```python
from build123d import *

# Parameters (mm, degrees)
SKETCH1_W           = 30
SKETCH1_H           = 13.3
BOSS_EXTRUDE1_DEPTH = 10.75
SKETCH2_W           = 8
SKETCH2_H           = 4.6
CUT_EXTRUDE1_DEPTH  = 6
FILLET1_R           = 0.2


with BuildPart() as part:
    # Sketch1 → Boss-Extrude1 (new body)
    with BuildSketch(Plane.XY):
        Rectangle(SKETCH1_W, SKETCH1_H)
    extrude(amount=BOSS_EXTRUDE1_DEPTH)

    # Sketch2 → Cut-Extrude1 (cut)
    with BuildSketch(Plane(origin=(15, 0, 0), x_dir=(0, 0, -1), z_dir=(1, 0, 0))):
        with Locations((-6.75, -3)):
            Rectangle(SKETCH2_W, SKETCH2_H)
        with Locations((-6.75, 3)):
            Rectangle(SKETCH2_W, SKETCH2_H)
    extrude(amount=-CUT_EXTRUDE1_DEPTH, mode=Mode.SUBTRACT)

    # Fillet1
    fillet1_edges = [part.edges().sort_by_distance(p)[0] for p in [
        (15, -5.975, 10.75),
        (15, 0, 10.75),
        (15, 5.975, 10.75),
        (0, 6.65, 10.75),
        (-15, 0, 10.75),
        (0, 6.65, 0),
        (15, 0, 0),
        (0, -6.65, 0),
        (-15, 0, 0),
        (-15, 6.65, 5.375),
        (15, 6.65, 5.375),
        (15, -6.65, 5.375),
        (-15, -6.65, 5.375),
        (0, -6.65, 10.75),
    ]]
    fillet(fillet1_edges, radius=FILLET1_R)


solid = part.part
```
Source: CAD feature listing. Evaluate the final solid. Frame: model axes, mm. A direction names the side the tool comes from. Give positions to 0.01 mm unless a question says otherwise; leave off trailing zeros. Loops run counter-clockwise (first coordinate to the right, second up) from the corner with the lowest first, then second, coordinate; pieces in that order, holes last. Notation, with made-up numbers: (89, 73) - (134, 73) arc R21 cw to (134, 84) - close; hole circle Ø6 at (80.5, 17.5). An arc over 180 degrees is marked (long way). Use CSV: the item, a comma, the result in double quotes. Start each with the question number.
1. Draft query along Y for faces 3 (the flat face through (15, 0, 4)), 4 (the flat face through (0, 6.65, 5)), 5 (the flat face through (12, 5.3, 7)). Return one class per face: +Y half, -Y half, draft (parallel to the pull), parting line (faces both ways), or undercut.
2. Section A-A (x = 10.5). Output: boundary loops of the cut face in (y, z).
3. Ray query, L1, parallel to X at y = -1.5, z = 10; L2, parallel to Z at x = 11, y = 1.25. Return the intervals inside material, ascending.
4. Section C-C (z = 9.5). Output: boundary loops of the cut face in (x, y), then the cut area to 3 significant figures.
5. Section B-B (y = -1.5). Output: boundary loops of the cut face in (x, z), then the cut area to 3 significant figures.
6. Reachability of faces 1 (the flat face through (0, -6.65, 5)), 2 (the flat face through (12, 0.7, 7)) from +Z, -Z, +X, -X, +Y, -Y: full face, straight path, thin tool, end or side. Return the list, or none.
7. Pin query (flat end, axial travel): pin 1 (6 mm diameter, centred on x = 10.5, y = 4, fed in from +Z); pin 2 (3.5 mm diameter, centred on x = 13, y = 3.5, fed in from +Z); pin 3 (3.5 mm diameter, centred on y = 2.5, z = 6, fed in from +X). Return the tip coordinate at first contact, or that it passes through.
Response:
1,face 3,"draft"
1,face 4,"+Y half"
1,face 5,"undercut"
2,outline,"(-6.65, 0.2) arc R0.2 ccw to (-6.45, 0) - (6.45, 0) arc R0.2 ccw to (6.65, 0.2) - (6.65, 10.55) arc R0.2 ccw to (6.45, 10.75) - (5.3, 10.75) - (5.3, 2.75) - (0.7, 2.75) - (0.7, 10.75) - (-0.7, 10.75) - (-0.7, 2.75) - (-5.3, 2.75) - (-5.3, 10.75) - (-6.45, 10.75) arc R0.2 ccw to (-6.65, 10.55) - close"
3,L1,"-15 to 9"
3,L2,"0 to 2.75"
4,outline,"(-15, -6.45) arc R0.2 ccw to (-14.8, -6.65) - (14.8, -6.65) arc R0.2 ccw to (15, -6.45) - (15, -5.3) - (9, -5.3) - (9, -0.7) - (15, -0.7) - (15, 0.7) - (9, 0.7) - (9, 5.3) - (15, 5.3) - (15, 6.45) arc R0.2 ccw to (14.8, 6.65) - (-14.8, 6.65) arc R0.2 ccw to (-15, 6.45) - close"
4,area,"344 mm²"
5,outline,"(-15, 0.2) arc R0.2 ccw to (-14.8, 0) - (14.8, 0) arc R0.2 ccw to (15, 0.2) - (15, 2.75) - (9, 2.75) - (9, 10.75) - (-14.8, 10.75) arc R0.2 ccw to (-15, 10.55) - close"
5,area,"274 mm²"
6,face 1,"+Z, -Z, +X, -X, -Y"
6,face 2,"+Z, +X"
7,pin 1,"z = 10.75"
7,pin 2,"z = 2.75"
7,pin 3,"x = 9"
